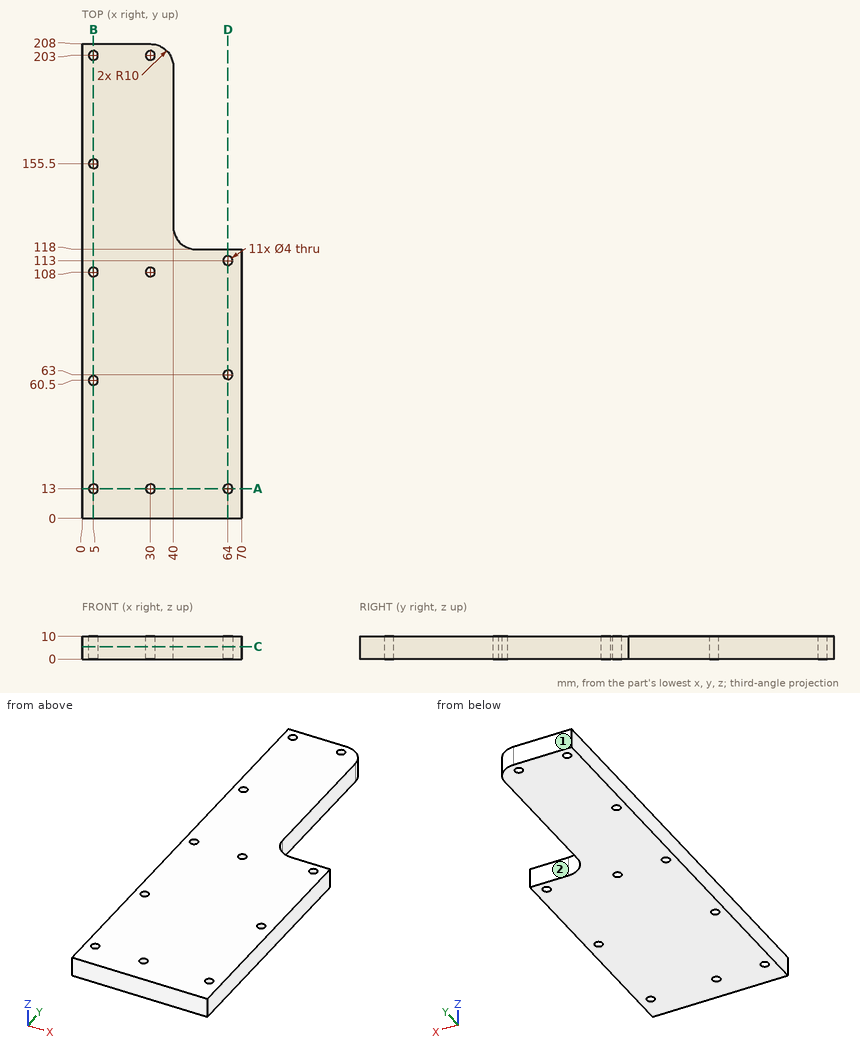
Job drawing, mm, ordinate dimensions from the low corner. One solid piece. A direction names the side the tool comes from. Coordinates: 2 decimals unless noted, no trailing zeros. Write each loop counter-clockwise with the first axis right and the second up, starting at its lowest first coordinate (ties: lowest second). Pieces come first, ordered by that corner, then holes. Notation, with made-up numbers: M 28.25,-17 L 70.25,-17 A7 cw 70.25,-12 Z; hole C -6.5,-29.5 d8. An arc over 180 degrees is marked long. Answer as a JSON object with one key per item and string values. Group by question number.
1) Tool access for the marked faces 1 and 2: list every direction of +Z, -Z, +X, -X, +Y, -Y with a clear straight run to the whole face (end or side of a thin tool).
2) Saw through at A-A (y = 13). Write the cut outline in (x, z).
3) Pin check, flat tips, straight feed: pin 1 Ø3 at (y, z) = (156, 2.5) entering from +X; pin 2 Ø3 at (x, y) = (5, 13) entering from +Z; pin 3 Ø3 at (x, z) = (59, 3) entering from +Y. Stop position of each tip, or through.
4) Wall check: line 1 (Y direction, x = 64, z = 3.5); line 2 (Y direction, x = 30, z = 6.75); line 3 (X direction, y = 106.5, z = 4.25). Give the ranges that are in metal, low to high. Write a range as from..to.
5) Saw through at C-C (z = 5.5). Give the number of separate pieces and of enclosed holes in the cut face, plus the area to 3 significant figures.
6) Saw through at B-B (x = 5). Write the cut outline in (y, z).
7) Saw through at D-D (x = 64). Write the cut outline in (y, z).
Values follow:
{
 "1": {"face 1": "+Z, -Z, +X, -X, +Y", "face 2": "+Z, -Z, +X, +Y"},
 "2": {"outline": "M 0,0 L 3,0 L 3,10 L 0,10 Z; M 7,0 L 28,0 L 28,10 L 7,10 Z; M 32,0 L 62,0 L 62,10 L 32,10 Z; M 66,0 L 70,0 L 70,10 L 66,10 Z"},
 "3": {"pin 1": "stops at x = 40", "pin 2": "passes through", "pin 3": "stops at y = 118"},
 "4": {"line 1": "y = 0..11, 15..61, 65..111, 115..118", "line 2": "y = 0..11, 15..106, 110..201, 205..208", "line 3": "x = 0..3.68, 6.32..28.68, 31.32..70"},
 "5": {"separate pieces": "1", "enclosed holes": "11", "area": "11,700 mm2"},
 "6": {"outline": "M 0,0 L 11,0 L 11,10 L 0,10 Z; M 15,0 L 58.5,0 L 58.5,10 L 15,10 Z; M 62.5,0 L 106,0 L 106,10 L 62.5,10 Z; M 110,0 L 153.5,0 L 153.5,10 L 110,10 Z; M 157.5,0 L 201,0 L 201,10 L 157.5,10 Z; M 205,0 L 208,0 L 208,10 L 205,10 Z"},
 "7": {"outline": "M 0,0 L 11,0 L 11,10 L 0,10 Z; M 15,0 L 61,0 L 61,10 L 15,10 Z; M 65,0 L 111,0 L 111,10 L 65,10 Z; M 115,0 L 118,0 L 118,10 L 115,10 Z"}
}
